Can you work these out from the drawing? Everything is in mm from the part's minimum corner. Give positions to 0.01 mm unless a question says otherwise; leave off trailing zeros. Loops run counter-clockwise (first coordinate to the right, second up) from the corner with the lowest first, then second, coordinate; pieces in that order, holes last. Notation, with made-up numbers: (3.25, -22.5) - (40.25, -22.5) arc R21 ccw to (40.25, -16.5) - close; hole circle Ø4 at (79, -3.75). An arc over 180 degrees is marked (long way). Answer in a Markdown table with one row per item.
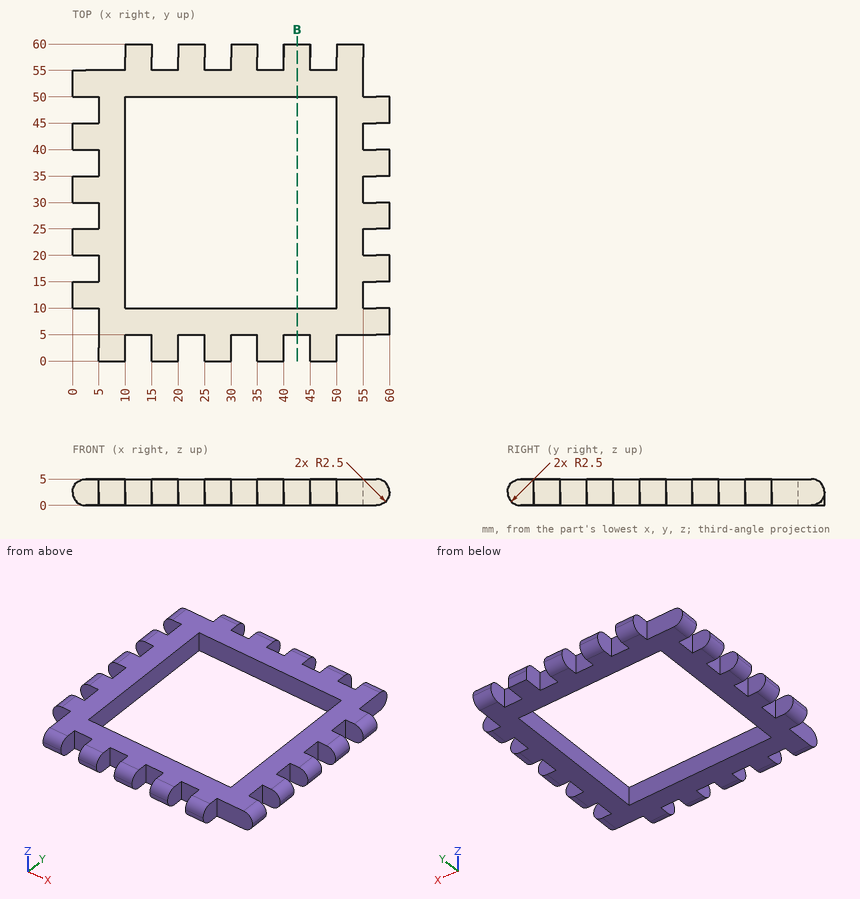
Q1. Imagine slicing it at B-B, the plane x = 42.5. Write out the boundary of the cut face in (y, z).
Checked values:
| item | result |
|---|---|
| outline | (5, 0) - (10, 0) - (10, 5) - (5, 5) - close; (50, 0) - (60, 0) - (60, 2.5) arc R2.5 ccw to (57.5, 5) - (50, 5) - close |
Q2. For pin 1 (2.5 mm diameter, centred on y = 3, z = 3.5, fed in from +X); pin 2 (2.5 mm diameter, centred on y = 48, z = 2, fed in from -X); pin 3 (2.5 mm diameter, centred on x = 2, z = 3.5, fed in from -Y), each with a flat end and sliding along its axis, tell me the tip position at first contact or that it passes through.
Checked values:
| item | result |
|---|---|
| pin 1 | stops at x = 50 |
| pin 2 | stops at x = 5 |
| pin 3 | stops at y = 10 |
Q3. If I drill on line 1 (Y direction, x = 57.5, z = 2.1); line 2 (Y direction, x = 46, z = 2.25); line 3 (X direction, y = 38.5, z = 2.4), over which ranges is the centre line in solid material (lowest first)? Write a range as [from, to].
Checked values:
| item | result |
|---|---|
| line 1 | y = [5, 10], [15, 20], [25, 30], [35, 40], [45, 50] |
| line 2 | y = [0.01, 10], [50, 55] |
| line 3 | x = [5, 10], [50, 60] |
